Source: CAD feature listing. Evaluate the final solid. Frame: model axes, mm. A direction names the side the tool comes from. Give positions to 0.01 mm unless a question says otherwise; leave off trailing zeros. Loops run counter-clockwise (first coordinate to the right, second up) from the corner with the lowest first, then second, coordinate; pieces in that order, holes last.
Autodesk Inventor part; units mm, degrees
ref_plane "YZ Plane" through (0, 0, 0) normal (1, 0, 0) x (0, 1, 0)
ref_plane "XZ Plane" through (0, 0, 0) normal (0, 1, 0) x (-1, 0, 0)
ref_plane "XY Plane" through (0, 0, 0) normal (0, 0, 1) x (1, 0, 0)
sketch "Boceto1" plane through (0, 0, 0) normal (0, 0, 1) x (1, 0, 0)
  line L0 (35, 35) -> (-35, 35) construction
  line L1 (-35, 35) -> (-35, -35) construction
  line L2 (-35, -35) -> (35, -35) construction
  line L3 (35, -35) -> (35, 35) construction
  circle A0 centre (35, 35) radius 2
  circle A1 centre (35, -35) radius 2
  circle A2 centre (-35, -35) radius 2
  circle A3 centre (-35, 35) radius 2
  circle A4 centre (0, 0) radius 32.5
  line L4 (50, 12) -> (50, -12)
  arc A5 (47.6827, -13.9747) -> (50, -12) centre (48, -12) ccw
  line L5 (47.6827, -13.9747) -> (40.6827, -12.85)
  arc A6 (39, -10.8753) -> (40.6827, -12.85) centre (41, -10.8753) ccw
  line L6 (39, -10.8753) -> (39, 10.8753)
  arc A7 (40.6827, 12.85) -> (39, 10.8753) centre (41, 10.8753) ccw
  line L7 (40.6827, 12.85) -> (47.6827, 13.9747)
  arc A8 (50, 12) -> (47.6827, 13.9747) centre (48, 12) ccw
  line L8 (0, 7) -> (32, 7) construction
  line L9 (32, 7) -> (32, 31) construction
  line L10 (32, 31) -> (0, 31) construction
  line L11 (0, 31) -> (0, 7) construction
  line L12 (29.5, -31) -> (29.5, -12) construction
  line L13 (29.5, -12) -> (2.5, -12) construction
  line L14 (2.5, -12) -> (2.5, -31) construction
  line L15 (2.5, -31) -> (29.5, -31) construction
  arc A9 (-37.5, -47.6) -> (-37.5, -43.4) centre (-37.5, -45.5) ccw
  arc A10 (-43.4, -37.5) -> (-37.5, -43.4) centre (-37.5, -37.5) ccw
  arc A11 (-43.4, -37.5) -> (-47.6, -37.5) centre (-45.5, -37.5) ccw
  arc A12 (-47.6, -37.5) -> (-37.5, -47.6) centre (-37.5, -37.5) ccw
  arc A13 (-47.6, 37.5) -> (-43.4, 37.5) centre (-45.5, 37.5) ccw
  arc A14 (-37.5, 43.4) -> (-43.4, 37.5) centre (-37.5, 37.5) ccw
  arc A15 (-37.5, 43.4) -> (-37.5, 47.6) centre (-37.5, 45.5) ccw
  arc A16 (-37.5, 47.6) -> (-47.6, 37.5) centre (-37.5, 37.5) ccw
  arc A17 (37.5, 47.6) -> (37.5, 43.4) centre (37.5, 45.5) ccw
  arc A18 (43.4, 37.5) -> (37.5, 43.4) centre (37.5, 37.5) ccw
  arc A19 (43.4, 37.5) -> (47.6, 37.5) centre (45.5, 37.5) ccw
  arc A20 (47.6, 37.5) -> (37.5, 47.6) centre (37.5, 37.5) ccw
  arc A21 (37.5, -43.4) -> (37.5, -47.6) centre (37.5, -45.5) ccw
  arc A22 (37.5, -47.6) -> (47.6, -37.5) centre (37.5, -37.5) ccw
  arc A23 (47.6, -37.5) -> (43.4, -37.5) centre (45.5, -37.5) ccw
  arc A24 (37.5, -43.4) -> (43.4, -37.5) centre (37.5, -37.5) ccw
  line L16 (-58.5, 20) -> (-58.5, -20)
  line L17 (-54.5, 20) -> (-58.5, 20)
  arc A25 (-54.5, 20) -> (-54.5, 24) centre (-54.5, 22) ccw
  line L18 (-54.5, 46.5) -> (-54.5, 24)
  line L19 (-46.5, 54.5) -> (-54.5, 46.5)
  line L20 (-24, 54.5) -> (-46.5, 54.5)
  arc A26 (-24, 54.5) -> (-20, 54.5) centre (-22, 54.5) ccw
  line L21 (-20, 58.5) -> (-20, 54.5)
  line L22 (20, 58.5) -> (-20, 58.5)
  line L23 (20, 54.5) -> (20, 58.5)
  arc A27 (20, 54.5) -> (24, 54.5) centre (22, 54.5) ccw
  line L24 (46.5, 54.5) -> (24, 54.5)
  line L25 (54.5, 46.5) -> (46.5, 54.5)
  line L26 (54.5, 24) -> (54.5, 46.5)
  arc A28 (54.5, 24) -> (54.5, 20) centre (54.5, 22) ccw
  line L27 (58.5, 20) -> (54.5, 20)
  line L28 (58.5, -20) -> (58.5, 20)
  line L29 (54.5, -20) -> (58.5, -20)
  arc A29 (54.5, -20) -> (54.5, -24) centre (54.5, -22) ccw
  line L30 (54.5, -46.5) -> (54.5, -24)
  line L31 (46.5, -54.5) -> (54.5, -46.5)
  line L32 (24, -54.5) -> (46.5, -54.5)
  arc A30 (24, -54.5) -> (20, -54.5) centre (22, -54.5) ccw
  line L33 (20, -58.5) -> (20, -54.5)
  line L34 (-20, -58.5) -> (20, -58.5)
  line L35 (-20, -54.5) -> (-20, -58.5)
  arc A31 (-20, -54.5) -> (-24, -54.5) centre (-22, -54.5) ccw
  line L36 (-46.5, -54.5) -> (-24, -54.5)
  line L37 (-54.5, -46.5) -> (-46.5, -54.5)
  line L38 (-54.5, -24) -> (-54.5, -46.5)
  arc A32 (-54.5, -24) -> (-54.5, -20) centre (-54.5, -22) ccw
  line L39 (-58.5, -20) -> (-54.5, -20)
  point P0 (35, 0)
  point P1 (58.5, 0)
  point P2 (0, 35)
  point P3 (39, 0)
  point P4 (50, 0)
  dimension "d0" = 70
  dimension "d1" = 4
  dimension "d2" = 65
  dimension "d3" = 2
  dimension "d4" = 11
  dimension "d5" = 28
  dimension "d6" = 25.7
  dimension "d8" = 4
extrude "Extrusión1" add sketch "Boceto1" along normal blind 4
properties part number "tapa ventilador"
(1) Section C-C, the plane y = 39. Return the cut outline in (x, z).
A:
outline: (-54.5, 0) - (-47.49, 0) - (-47.49, 4) - (-54.5, 4) - close; (-43.21, 0) - (43.21, 0) - (43.21, 4) - (-43.21, 4) - close; (47.49, 0) - (54.5, 0) - (54.5, 4) - (47.49, 4) - close
(2) Section B-B, the plane y = -17.5. Return the cut outline in (x, z).
A:
outline: (-58.5, 0) - (-27.39, 0) - (-27.39, 4) - (-58.5, 4) - close; (27.39, 0) - (58.5, 0) - (58.5, 4) - (27.39, 4) - close
(3) Reachability of faces 4 (the flat face through (-35, 54.5, 2)), 5 (the cylindrical face through (-35.4, -45.5, 2)), 6 (the flat face through (54.5, 35, 2)) from +Z, -Z, +X, -X, +Y, -Y: full face, straight path, thin tool, end or side. Return the list, or none.
A:
face 4: +Z, -Z, -X, +Y
face 5: +Z, -Z
face 6: +Z, -Z, +X, +Y
(4) First-contact query: pin 1 (1.2 mm diameter, centred on y = 31.5, z = 1.5, fed in from -X); pin 2 (2 mm diameter, centred on x = 35, z = 1.5, fed in from +Y); pin 3 (1.2 mm diameter, centred on x = 32.5, z = 1.5, fed in from -Y). Flat tips, straight axial feed; report the tip coordinate or a pass-through.
A:
pin 1: stops at x = -54.5
pin 2: stops at y = 54.5
pin 3: stops at y = -54.5
(5) Ray query, line 1 along Y through (x, z) = (-35, 2.4); line 2 along Y through (x, z) = (-38, 2); line 3 along X through (y, z) = (-42, 3.1). Return the intervals inside material, ascending.
A:
line 1: y = -54.5 to -37, -33 to 33, 37 to 54.5
line 2: y = -54.5 to -47.59, -43.38 to 43.38, 47.59 to 54.5
line 3: x = -54.5 to -46.54, -41.32 to 41.32, 46.54 to 54.5
(6) Section D-D, the plane z = 3.3. Count the separate pieces of the cut face and the enclosed holes in it, then the cut area to 3 significant figures.
A:
separate pieces: 1
enclosed holes: 10
area: 8,420 mm2
(7) Section A-A, the plane x = 0. Return the cut outline in (y, z).
A:
outline: (-58.5, 0) - (-32.5, 0) - (-32.5, 4) - (-58.5, 4) - close; (32.5, 0) - (58.5, 0) - (58.5, 4) - (32.5, 4) - close
(8) Mould query, pull axis X, two halves, no side actions, for faces 1 (the flat face through (51, 50, 2)), 2 (the flat face through (25, -25, 0)), 3 (the flat face through (39, 0, 2)). Classes: pulls with the +X half, pulls with the -X half, needs draft (parallel to the pull), parting line crosses it, or undercut.
A:
face 1: pulls with the +X half
face 2: needs draft
face 3: undercut
